Could you check a few things on this model? Use its own coordinates, in mm. Face numbers are marked on the shaded views. Give positions to 0.01 mm unless a question says otherwise; leave off trailing zeros. Loops run counter-clockwise (first coordinate to the right, second up) from the corner with the lowest first, then second, coordinate; pieces in that order, holes last. Notation, with made-up numbers: (44, -24.5) -> (91, -24.5) arc R17 cw to (91, -9.5) -> close; hole circle Ø6 at (58.25, 8). An arc over 180 degrees is marked (long way). Put each result on its own line as item: value.
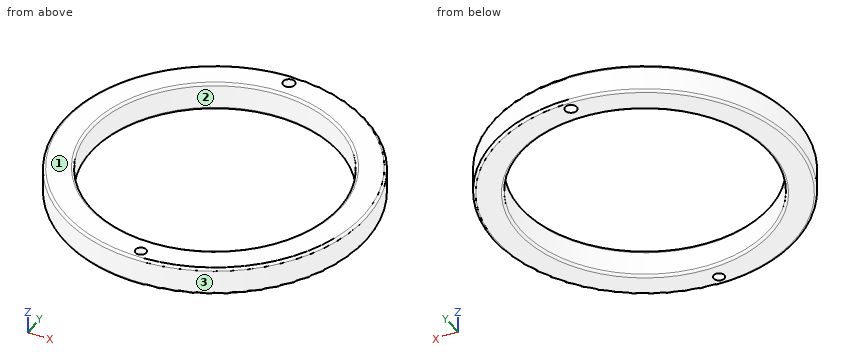
```python
from build123d import *

# Parameters (mm, degrees)
F0_R     = 31.75
F0_R_2   = 1.125
F0_R_3   = 26
F0_R_4   = 1.225
F1_DEPTH = 5
F2_DEPTH = 5.9
F3_R     = 0.5
F4_R     = 0.5


with BuildPart() as f1:
    # F0 (on Top) → F1 (new body)
    with BuildSketch(Plane.XY):
        Circle(F0_R)
        with Locations((0, -29.5)):
            Circle(F0_R_2, mode=Mode.SUBTRACT)
        Circle(F0_R_3, mode=Mode.SUBTRACT)
        with Locations((0, 29.5)):
            Circle(F0_R_4, mode=Mode.SUBTRACT)
    extrude(amount=F1_DEPTH)

    # F0 (on Top) → F2 (join)
    with BuildSketch(Plane.XY):
        Circle(F0_R)
        with Locations((0, -29.5)):
            Circle(F0_R_2, mode=Mode.SUBTRACT)
        Circle(F0_R_3, mode=Mode.SUBTRACT)
        with Locations((0, 29.5)):
            Circle(F0_R_4, mode=Mode.SUBTRACT)
    extrude(amount=F2_DEPTH)

    # F3
    f3_edges = [f1.edges().sort_by_distance(p)[0] for p in [
        (-26, 0, 0),
        (-31.75, 0, 0),
        (-31.75, 0, 5.9),
    ]]
    fillet(f3_edges, radius=F3_R)

    # F4
    f4_edges = [f1.edges().sort_by_distance(p)[0] for p in [
        (-26, 0, 5.9),
        (-31.75, 0, 5.4),
    ]]
    fillet(f4_edges, radius=F4_R)


solid = f1.part
```
1. Thinking about a two-plate mould opening in X: for the marked faces 1, 2 and 3, which applies, pulls with the +X half, pulls with the -X half, needs draft (parallel to the pull), parting line crosses it, or undercut?
Recorded:
face 1: needs draft
face 2: undercut
face 3: parting line crosses it
2. If we section it at B-B (x = 0): List the corners of the cut face in (y, z) for me (3 decimals), then the cut area to 3 significant figures.
Recorded:
outline: (-31.75, 0.5) arc R0.5 ccw to (-31.25, 0) -> (-30.625, 0) -> (-30.625, 5.9) -> (-31.25, 5.9) arc R0.5 ccw to (-31.75, 5.4) -> close; (-28.375, 0) -> (-26.5, 0) arc R0.5 ccw to (-26, 0.5) -> (-26, 5.4) arc R0.5 ccw to (-26.5, 5.9) -> (-28.375, 5.9) -> close; (26, 0.5) arc R0.5 ccw to (26.5, 0) -> (28.275, 0) -> (28.275, 5.9) -> (26.5, 5.9) arc R0.5 ccw to (26, 5.4) -> close; (30.725, 0) -> (31.25, 0) arc R0.5 ccw to (31.75, 0.5) -> (31.75, 5.4) arc R0.5 ccw to (31.25, 5.9) -> (30.725, 5.9) -> close
area: 39.7 mm^2
3. If we section it at A-A (y = 0): List the corners of the cut face in (x, z) for me, then the cut area to 3 significant figures.
Recorded:
outline: (-31.75, 0.5) arc R0.5 ccw to (-31.25, 0) -> (-26.5, 0) arc R0.5 ccw to (-26, 0.5) -> (-26, 5.4) arc R0.5 ccw to (-26.5, 5.9) -> (-31.25, 5.9) arc R0.5 ccw to (-31.75, 5.4) -> close; (26, 0.5) arc R0.5 ccw to (26.5, 0) -> (31.25, 0) arc R0.5 ccw to (31.75, 0.5) -> (31.75, 5.4) arc R0.5 ccw to (31.25, 5.9) -> (26.5, 5.9) arc R0.5 ccw to (26, 5.4) -> close
area: 67.4 mm^2
4. If we section it at C-C (z = 3.7): List the corners of the cut face in (x, y) for me (3 decimals).
Recorded:
outline: circle Ø63.5 at (0, 0); hole circle Ø52 at (0, 0); hole circle Ø2.45 at (0, 29.5); hole circle Ø2.25 at (0, -29.5)
5. I'm going to push flat-ended pins straight in: pin 1 (3 mm diameter, centred on x = 8, z = 3, fed in from +Y); pin 2 (1 mm diameter, centred on x = -14.5, z = 4.5, fed in from +Y); pin 3 (3 mm diameter, centred on x = 20.5, z = 5, fed in from -Y). Where does each tip first touch, or does it pass through?
Recorded:
pin 1: stops at y = 31.08
pin 2: stops at y = 28.5
pin 3: stops at y = -25.44
6. I need wall thicknesses on line 1 (Y direction, x = 0, z = 3.1) (3 decimals); line 2 (X direction, y = -0.5, z = 3.15); line 3 (Y direction, x = 1, z = 5.45). Which ranges of each line are inside material? Lowest first, please.
Recorded:
line 1: y = -31.75 to -30.625, -28.375 to -26, 26 to 28.275, 30.725 to 31.75
line 2: x = -31.75 to -26, 26 to 31.75
line 3: y = -31.73 to -30.02, -28.98 to -25.98, 25.98 to 28.79, 30.21 to 31.73
